Design review of the part built by this model. Coordinates are the model's own, in mm. Give positions to 0.01 mm unless a question says otherwise; leave off trailing zeros. Write each loop counter-clockwise with the first axis right and the second up, starting at its lowest first coordinate (ties: lowest second). Pieces come first, ordered by that corner, then holes. Notation, with made-up numbers: (-30, -19.75) -> (5, -19.75) arc R34 ccw to (5, 16.25) -> close; hole circle Ø1 at (-37.75, 37). An arc over 180 degrees is marked (long way). Use CSV: the item, a comma, the result in double quotes.
```python
from build123d import *

# Parameters (mm, degrees)
F0_R     = 12.6376963258
F1_DEPTH = 10.16
F2_R     = 5.07999
F3_R     = 2.5783631355
F4_DEPTH = 25.4


# Not quite as in the source:
# - a fillet or chamfer is up to 0.001 mm smaller than in the source, because OpenCascade refuses the exact size


with BuildPart() as f1:
    # F0 (on Front) → F1 (new body)
    with BuildSketch(Plane.XZ):
        with Locations((-57.7037265382, 0)):
            Circle(F0_R)
    extrude(amount=F1_DEPTH)

    # F2 (radius 5.08 in the source; OpenCascade refuses exactly that, so slightly less here)
    f2_edges = [f1.edges().sort_by_distance(p)[0] for p in [
        (-70.341423, 0, 0),
        (-70.341423, -10.16, 0),
    ]]
    fillet(f2_edges, radius=F2_R)

    # F3 (on Front) → F4 (cut)
    with BuildSketch(Plane.XZ):
        with Locations((-57.7121302485, 0)):
            Circle(F3_R)
    extrude(amount=F4_DEPTH, mode=Mode.SUBTRACT)


solid = f1.part
```
(1) Take a section at C-C (y = -7.5). Write out the cut boundary in (x, z), then the cut area to 3 significant figures.
Established:
outline,"circle Ø24.05 at (-57.7, 0); hole circle Ø5.16 at (-57.71, 0)"
area,"433 mm2"
(2) For line 1 along Z through (x, y) = (-57.5, -3); line 2 along Z through (x, y) = (-57, -4.75); line 3 along X through (y, z) = (-9, -2), list the stretches that pass through material, from the lowest coordinate up. Write a range as [from, to].
Established:
line 1,"z = [-12.19, -2.57], [2.57, 12.19]"
line 2,"z = [-12.61, -2.48], [2.48, 12.61]"
line 3,"x = [-68.31, -59.34], [-56.08, -47.1]"
(3) Clearance check with flat-ended pins moving along their axes: pin 1 (6 mm diameter, centred on y = -8.5, z = 8.5, fed in from -X); pin 2 (2 mm diameter, centred on x = -49.5, z = -10, fed in from -Y); pin 3 (1.5 mm diameter, centred on y = -2, z = -9, fed in from -X). State where each tip first meets the part, or that it passes through.
Established:
pin 1,"stops at x = -68.47"
pin 2,"stops at y = -7.66"
pin 3,"stops at x = -66.14"
(4) Mouldability with a two-part tool opening along Z and no side actions: class faces 1 (the face through (-60.29, -5.01, 0.11)), 2 (the face through (-58, 0, -3)) as +Z half, -Z half, draft (parallel to the pull), parting line (faces both ways), or undercut.
Established:
face 1,"undercut"
face 2,"draft"
(5) Take a section at B-B (y = -1.75). Write out the cut boundary in (x, z), then the cut area to 3 significant figures.
Established:
outline,"circle Ø22.79 at (-57.7, 0); hole circle Ø5.16 at (-57.71, 0)"
area,"387 mm2"
